Source: CAD feature listing. Evaluate the final solid. Frame: model axes, mm. A direction names the side the tool comes from. Give positions to 0.01 mm unless a question says otherwise; leave off trailing zeros. Write each loop counter-clockwise with the first axis right and the second up, starting at its lowest first coordinate (ties: lowest second). Pieces come first, ordered by that corner, then holes. Notation, with made-up numbers: (33.5, 47) - (85.5, 47) arc R23 ccw to (85.5, 78) - close; hole circle Ø9 at (35, -12). An arc over 180 degrees is marked (long way). Answer as a JSON object with one key per item and string values. Group by question number.
from build123d import *

# Parameters (mm, degrees)
F0_R      = 25
F1_DEPTH  = 40
F2_R      = 2.5
F3_DEPTH  = 1
F5_DEPTH  = 40.001
F7_DEPTH  = 40
F8_R      = 2.5
F9_DEPTH  = 1
F10_R     = 1.5
F11_DEPTH = 5


with BuildPart() as f1:
    # F0 (on Front) → F1 (new body)
    with BuildSketch(Plane.XZ):
        Circle(F0_R)
    extrude(amount=F1_DEPTH)

    # F2 (on face) → F3 (cut)
    with BuildSketch(Plane(origin=(0, 0, 0), x_dir=(-1, 0, 0), z_dir=(0, 1, 0))):
        Circle(F2_R)
    extrude(amount=-F3_DEPTH, mode=Mode.SUBTRACT)

    # F4 (on face) → F5 (cut, through all)
    with BuildSketch(Plane(origin=(0, 0, 0), x_dir=(-1, 0, 0), z_dir=(0, 1, 0))):
        with BuildLine():
            ThreePointArc((8.1327834988, 9.4925145542), (10.1127124297, 7.3473156537), (11.5410861355, 4.8013884256))
            Line((11.5410861355, 4.8013884256), (23.4483671681, 8.6702985617))
            ThreePointArc((23.4483671681, 8.6702985617), (20.2254248594, 14.6946313073), (15.4918878906, 19.6214527899))
            Line((15.4918878906, 19.6214527899), (8.1327834988, 9.4925145542))
        make_face()
        with BuildLine():
            ThreePointArc((1, 12.4599357944), (3.8627124297, 11.8882064537), (6.5147495101, 10.6680850588))
            Line((6.5147495101, 10.6680850588), (13.8738539018, 20.7970232945))
            ThreePointArc((13.8738539018, 20.7970232945), (7.7254248594, 23.7764129074), (1, 24.9799919936))
            Line((1, 24.9799919936), (1, 12.4599357944))
        make_face()
        with BuildLine():
            ThreePointArc((-6.5147495101, 10.6680850588), (-3.8627124297, 11.8882064537), (-1, 12.4599357944))
            Line((-1, 12.4599357944), (-1, 24.9799919936))
            ThreePointArc((-1, 24.9799919936), (-7.7254248594, 23.7764129074), (-13.8738539018, 20.7970232945))
            Line((-13.8738539018, 20.7970232945), (-6.5147495101, 10.6680850588))
        make_face()
        with BuildLine():
            ThreePointArc((-11.5410861355, 4.8013884256), (-10.1127124297, 7.3473156537), (-8.1327834988, 9.4925145542))
            Line((-8.1327834988, 9.4925145542), (-15.4918878906, 19.6214527899))
            ThreePointArc((-15.4918878906, 19.6214527899), (-20.2254248594, 14.6946313073), (-23.4483671681, 8.6702985617))
            Line((-23.4483671681, 8.6702985617), (-11.5410861355, 4.8013884256))
        make_face()
        with BuildLine():
            ThreePointArc((-12.1591201242, -2.899275393), (-12.5, 0), (-12.1591201242, 2.899275393))
            Line((-12.1591201242, 2.899275393), (-24.0664011569, 6.7681855291))
            ThreePointArc((-24.0664011569, 6.7681855291), (-25, 0), (-24.0664011569, -6.7681855291))
            Line((-24.0664011569, -6.7681855291), (-12.1591201242, -2.899275393))
        make_face()
        with BuildLine():
            Line((-15.4918878906, -19.6214527899), (-8.1327834988, -9.4925145542))
            ThreePointArc((-8.1327834988, -9.4925145542), (-10.1127124297, -7.3473156537), (-11.5410861355, -4.8013884256))
            Line((-11.5410861355, -4.8013884256), (-23.4483671681, -8.6702985617))
            ThreePointArc((-23.4483671681, -8.6702985617), (-20.2254248594, -14.6946313073), (-15.4918878906, -19.6214527899))
        make_face()
        with BuildLine():
            Line((-1, -24.9799919936), (-1, -12.4599357944))
            ThreePointArc((-1, -12.4599357944), (-3.8627124297, -11.8882064537), (-6.5147495101, -10.6680850588))
            Line((-6.5147495101, -10.6680850588), (-13.8738539018, -20.7970232945))
            ThreePointArc((-13.8738539018, -20.7970232945), (-7.7254248594, -23.7764129074), (-1, -24.9799919936))
        make_face()
        with BuildLine():
            Line((13.8738539018, -20.7970232945), (6.5147495101, -10.6680850588))
            ThreePointArc((6.5147495101, -10.6680850588), (3.8627124297, -11.8882064537), (1, -12.4599357944))
            Line((1, -12.4599357944), (1, -24.9799919936))
            ThreePointArc((1, -24.9799919936), (7.7254248594, -23.7764129074), (13.8738539018, -20.7970232945))
        make_face()
        with BuildLine():
            Line((23.4483671681, -8.6702985617), (11.5410861355, -4.8013884256))
            ThreePointArc((11.5410861355, -4.8013884256), (10.1127124297, -7.3473156537), (8.1327834988, -9.4925145542))
            Line((8.1327834988, -9.4925145542), (15.4918878906, -19.6214527899))
            ThreePointArc((15.4918878906, -19.6214527899), (20.2254248594, -14.6946313073), (23.4483671681, -8.6702985617))
        make_face()
        with BuildLine():
            ThreePointArc((12.1591201242, 2.899275393), (12.4144875358, 1.4596229731), (12.5, 0))
            ThreePointArc((12.5, 0), (12.4144875358, -1.4596229731), (12.1591201242, -2.899275393))
            Line((12.1591201242, -2.899275393), (24.0664011569, -6.7681855291))
            ThreePointArc((24.0664011569, -6.7681855291), (24.7655004888, -3.4161360539), (25, 0))
            ThreePointArc((25, 0), (24.7655004888, 3.4161360539), (24.0664011569, 6.7681855291))
            Line((24.0664011569, 6.7681855291), (12.1591201242, 2.899275393))
        make_face()
    extrude(amount=-F5_DEPTH, mode=Mode.SUBTRACT)

    # F6 (on face) → F7 (join)
    with BuildSketch(Plane(origin=(0, 0, 0), x_dir=(-1, 0, 0), z_dir=(0, 1, 0))):
        with BuildLine():
            ThreePointArc((2.5, 0), (2.0225424859, 1.4694631307), (0.7725424859, 2.3776412907))
            ThreePointArc((0.7725424859, 2.3776412907), (-2.0225424859, -1.4694631307), (2.5, 0))
        make_face()
        with BuildLine():
            ThreePointArc((-3.1909113793, -12.0858630048), (-3.8627124297, -11.8882064537), (-4.5223905021, -11.6532392126))
            Line((-4.5223905021, -11.6532392126), (-6.2671362955, -17.0230146177))
            ThreePointArc((-6.2671362955, -17.0230146177), (-5.5623058987, -17.1190172933), (-4.9356571727, -17.4556384098))
            Line((-4.9356571727, -17.4556384098), (-3.1909113793, -12.0858630048))
        make_face()
        with BuildLine():
            Line((-6.5260565798, -17.819889314), (-6.2671362955, -17.0230146177))
            ThreePointArc((-6.2671362955, -17.0230146177), (-7.5635259169, -20.465705145), (-4.1803398875, -19.0211303259))
            ThreePointArc((-4.1803398875, -19.0211303259), (-4.379039603, -18.1520404081), (-4.9356571727, -17.4556384098))
            Line((-4.9356571727, -17.4556384098), (-5.194577457, -18.2525131061))
            ThreePointArc((-5.194577457, -18.2525131061), (-4.9982436481, -18.6147456794), (-4.9303398875, -19.0211303259))
            ThreePointArc((-4.9303398875, -19.0211303259), (-6.9321224806, -20.0197908952), (-6.5260565798, -17.819889314))
        make_face()
        with BuildLine():
            ThreePointArc((3.1909113793, 12.0858630048), (3.5281963151, 11.9917401057), (3.8627124297, 11.8882064537))
            Line((3.8627124297, 11.8882064537), (5.5623058987, 17.1190172933))
            ThreePointArc((5.5623058987, 17.1190172933), (5.233895582, 17.2592440706), (4.9356571727, 17.4556384098))
            Line((4.9356571727, 17.4556384098), (3.1909113793, 12.0858630048))
        make_face()
        with BuildLine():
            Line((5.5623058987, 17.1190172933), (3.8627124297, 11.8882064537))
            ThreePointArc((3.8627124297, 11.8882064537), (4.1941972051, 11.7753432988), (4.5223905021, 11.6532392126))
            Line((4.5223905021, 11.6532392126), (6.2671362955, 17.0230146177))
            ThreePointArc((6.2671362955, 17.0230146177), (5.9104186578, 17.0394283983), (5.5623058987, 17.1190172933))
        make_face()
        with BuildLine():
            ThreePointArc((6.7983738762, 20.9232433585), (4.4184536322, 19.9675746314), (4.9356571727, 17.4556384098))
            Line((4.9356571727, 17.4556384098), (5.194577457, 18.2525131061))
            ThreePointArc((5.194577457, 18.2525131061), (5.1567490659, 19.7385993706), (6.5666111305, 20.2099509713))
            Line((6.5666111305, 20.2099509713), (6.7983738762, 20.9232433585))
        make_face()
        with BuildLine():
            Line((6.5260565798, 17.819889314), (6.2671362955, 17.0230146177))
            ThreePointArc((6.2671362955, 17.0230146177), (7.6249147066, 17.6379442965), (8.1803398875, 19.0211303259))
            ThreePointArc((8.1803398875, 19.0211303259), (7.7983738762, 20.1967008305), (6.7983738762, 20.9232433585))
            Line((6.7983738762, 20.9232433585), (6.5666111305, 20.2099509713))
            ThreePointArc((6.5666111305, 20.2099509713), (7.1916111305, 19.7558618913), (7.4303398875, 19.0211303259))
            ThreePointArc((7.4303398875, 19.0211303259), (7.1790004568, 18.2693477328), (6.5260565798, 17.819889314))
        make_face()
        with BuildLine():
            ThreePointArc((-4.9356571727, -17.4556384098), (-5.5623058987, -17.1190172933), (-6.2671362955, -17.0230146177))
            Line((-6.2671362955, -17.0230146177), (-6.5260565798, -17.819889314))
            ThreePointArc((-6.5260565798, -17.819889314), (-5.7940686445, -17.8323096805), (-5.194577457, -18.2525131061))
            Line((-5.194577457, -18.2525131061), (-4.9356571727, -17.4556384098))
        make_face()
        with BuildLine():
            ThreePointArc((4.9356571727, 17.4556384098), (5.233895582, 17.2592440706), (5.5623058987, 17.1190172933))
            Line((5.5623058987, 17.1190172933), (5.7940686445, 17.8323096805))
            ThreePointArc((5.7940686445, 17.8323096805), (5.4628708429, 17.9975395043), (5.194577457, 18.2525131061))
            Line((5.194577457, 18.2525131061), (4.9356571727, 17.4556384098))
        make_face()
        with BuildLine():
            Line((5.7940686445, 17.8323096805), (5.5623058987, 17.1190172933))
            ThreePointArc((5.5623058987, 17.1190172933), (5.9104186578, 17.0394283983), (6.2671362955, 17.0230146177))
            Line((6.2671362955, 17.0230146177), (6.5260565798, 17.819889314))
            ThreePointArc((6.5260565798, 17.819889314), (6.1591329483, 17.7713102326), (5.7940686445, 17.8323096805))
        make_face()
    extrude(amount=-F7_DEPTH)

    # F8 (on face) → F9 (cut)
    with BuildSketch(Plane.XZ.offset(40)):
        Circle(F8_R)
    extrude(amount=-F9_DEPTH, mode=Mode.SUBTRACT)

    # F10 (on face) → F11 (cut)
    with BuildSketch(Plane(origin=(0, 0, 0), x_dir=(-1, 0, 0), z_dir=(0, 1, 0))):
        with Locations((10, 0)):
            Circle(F10_R)
        with Locations((-10, -0.6205414017)):
            Circle(F10_R)
        with Locations((0, -10)):
            Circle(F10_R)
        with Locations((0, 10)):
            Circle(F10_R)
    extrude(amount=-F11_DEPTH, mode=Mode.SUBTRACT)


solid = f1.part
Q1. Section B-B on y = -16. State how many separate pieces and enclosed holes the cut face has, then the cut area to 3 significant figures.
Q2. Draft query along Z for faces 1 (the cylindrical face through (11.5, -2.5, -0.6)), 2 (the cylindrical face through (-10.14, -19.72, -7.31)), 3 (the cylindrical face through (0, -20, -25)), 4 (the cylindrical face through (3.902, -19.72, 11.875)). Return one class per face: released by +Z, released by -Z, zero draft, split by the parting line, or undercut.
Q3. Section A-A on x = 10. Return the cut outline in (y, z), then the cut area to 3 significant figures.
Q4. Ray query, probe 1 along Z at (x, y) = (0, -3.35); probe 2 along Z at (x, y) = (-10, -1); probe 3 along Z at (x, y) = (-9, -26). Return the intervals inside material, ascending. Write a range as [from, to].
Q5. Section C-C on x = 0. Return the cut outline in (y, z), then the cut area to 4 significant figures.
Q6. Reachability of faces 5 (the flat face through (5.383, -19.72, -14.301)), 6 (the flat face through (10, -5, -1)), 7 (the flat face through (-1, -20, 19)) from +Z, -Z, +X, -X, +Y, -Y: full face, straight path, thin tool, end or side. Return the list, or none.
Q7. First-contact query: pin 1 Ø10 at (y, z) = (-14, 20) entering from +X; pin 2 Ø5 at (y, z) = (-33, 14) entering from -X; pin 3 Ø1.5 at (x, z) = (-0.5, -9.5) entering from +Y. Flat tips, straight axial feed; report the tip coordinate or a pass-through.
Taken from the geometry:
{
 "1": {"separate pieces": "1", "enclosed holes": "2", "area": "772 mm²"},
 "2": {"face 1": "undercut", "face 2": "undercut", "face 3": "released by -Z", "face 4": "released by +Z"},
 "3": {"outline": "(-40, -15.47) - (0, -15.47) - (0, -12.06) - (-40, -12.06) - close; (-40, -7.5) - (0, -7.5) - (0, -2.12) - (-5, -2.12) - (-5, 0.88) - (0, 0.88) - (0, 7.5) - (-40, 7.5) - close; (-40, 12.06) - (0, 12.06) - (0, 15.47) - (-40, 15.47) - close", "area": "857 mm²"},
 "4": {"probe 1": "z = [-25, -11.5], [-8.5, 8.5], [11.5, 25]", "probe 2": "z = [-15.47, -12.06], [-7.5, -1.5], [1.5, 7.5], [12.06, 15.47]", "probe 3": "z = [-14.09, -10.69], [-8.67, 8.67], [10.69, 14.09]"},
 "5": {"outline": "(-40, -25) - (0, -25) - (0, -11.5) - (-5, -11.5) - (-5, -8.5) - (0, -8.5) - (0, 8.5) - (-5, 8.5) - (-5, 11.5) - (0, 11.5) - (0, 25) - (-40, 25) - (-40, 2.5) - (-39, 2.5) - (-39, -2.5) - (-40, -2.5) - close", "area": "1,965 mm²"},
 "6": {"face 5": "+Y, -Y", "face 6": "+Y", "face 7": "+Z, +Y, -Y"},
 "7": {"pin 1": "stops at x = 15.49", "pin 2": "stops at x = -13.22", "pin 3": "stops at y = -5"}
}
